Source: CAD feature listing. Evaluate the final solid. Frame: model axes, mm. A direction names the side the tool comes from. Give positions to 0.01 mm unless a question says otherwise; leave off trailing zeros. Order: outer loops, then holes, each group sorted by start corner. A loop starts at its lowest first (then second) coordinate and runs counter-clockwise, first axis right, second up.
1) Material intervals for line 1 (X direction, y = 3.75, z = 43); line 2 (X direction, y = 3, z = 8.5); line 3 (Z direction, x = 40.5, y = 27.25), sorted ascending.
2) Section C-C, the plane x = 43.5. Return loops of the section in (y, z), plus the area to 3 significant figures.
3) Section B-B, the plane z = 20. Return loops of the section in (x, y).
4) First-contact query: P1, Ø3, axis at y = 13.5, z = 16.5, coming from the +X side; P2, Ø2, axis at y = 13.5, z = 23.5, coming from the -X side; P3, Ø1, axis at x = 58, y = 11.5, coming from the -Z side; P4, Ø10, axis at y = 6.5, z = 9, coming from the -X side. Flat tips, straight axial feed; report the tip coordinate or a pass-through.
5) Access query for faces 1 (the face through (53, 23, 28.7)), 2 (the face through (60.25, 14, -2)), 3 (the face through (49.25, 14, 22)), 4 (the face through (21.75, 5, 27)). Directions: +Z, -Z, +X, -X, +Y, -Y. A direction counts if a zero-diameter tool reaches every point of the face in a straight line with its end or side. Return the directions, or none.
6) Section D-D, the plane x = 62. Return loops of the section in (y, z).
7) Draft query along X for faces 5 (the face through (49.25, 5, 27)), 6 (the face through (60.25, 5, 22)), 7 (the face through (55, 10.7, 23)). Return one class per face: released by +X, released by -X, zero draft, split by the parting line, or undercut.
8) Section A-A, the plane y = 6.5. Return loops of the section in (x, z), plus the area to 3 significant figures.
```python
from build123d import *

# Parameters (mm, degrees)
F0_W     = 10.75
F0_H     = 8.6
F1_DEPTH = 3.3
F0_W_2   = 27
F0_H_2   = 21
F0_W_3   = 7.25
F0_H_3   = 10.7
F0_H_4   = 6.6
F0_W_4   = 3.75
F2_DEPTH = 4.7
F3_DEPTH = 17.5
F4_DEPTH = 28.7
F5_DEPTH = 26
F6_DEPTH = 61.5
F7_SIZE  = 3
F8_R     = 1.5


with BuildPart() as f1:
    # F0 (on Top) → F1 (new body)
    with BuildSketch(Plane.XY):
        Polygon((-3.5, 0), (0, 0), (0, 8.6), (0, 9), (-3.5, 9), align=None)
        with Locations((5.375, 4.3)):
            Rectangle(F0_W, F0_H)
        Polygon((0, 9), (0, 8.6), (10.75, 8.6), (10.75, 10.7), (10.75, 17.3), (10.75, 28), (0, 28), (0, 19), align=None)
    extrude(amount=-F1_DEPTH)



with BuildPart() as f1b:
    # F0 (on Top) → F1, piece 2 (new body)
    with BuildSketch(Plane.XY):
        Polygon((71, 19.4), (71, 19), (74.5, 19), (74.5, 28), (71, 28), align=None)
        with Locations((65.625, 23.7)):
            Rectangle(F0_W, F0_H)
        Polygon((60.25, 10.7), (60.25, 0), (71, 0), (71, 9), (71, 19), (71, 19.4), (60.25, 19.4), (60.25, 17.3), align=None)
    extrude(amount=-F1_DEPTH)


with BuildPart() as f1_1:
    add(f1.part)

    add(f1b.part)  # F2 merges F1b
    # F0 (on Top) → F2 (join)
    with BuildSketch(Plane.XY):
        Polygon((21.75, 10.7), (21.75, 0), (49.25, 0), (49.25, 10.7), (49.25, 17.3), (49.25, 28), (21.75, 28), (21.75, 17.3), align=None)
        with Locations((35.5, 14)):
            Rectangle(F0_W_2, F0_H_2, mode=Mode.SUBTRACT)
        with Locations((35.5, 14)):
            Rectangle(F0_W_2, F0_H_2)
        Polygon((0, 9), (0, 8.6), (10.75, 8.6), (10.75, 10.7), (10.75, 17.3), (10.75, 28), (0, 28), (0, 19), align=None)
        Polygon((60.25, 10.7), (60.25, 0), (71, 0), (71, 9), (71, 19), (71, 19.4), (60.25, 19.4), (60.25, 17.3), align=None)
        with Locations((65.625, 23.7)):
            Rectangle(F0_W, F0_H)
        with Locations((5.375, 4.3)):
            Rectangle(F0_W, F0_H)
        with Locations((56.625, 5.35)):
            Rectangle(F0_W_3, F0_H_3)
        Polygon((53, 28), (53, 17.3), (60.25, 17.3), (60.25, 19.4), (60.25, 28), align=None)
        Polygon((10.75, 8.6), (10.75, 0), (18, 0), (18, 10.7), (10.75, 10.7), align=None)
        with Locations((14.375, 22.65)):
            Rectangle(F0_W_3, F0_H_3)
        with Locations((14.375, 14)):
            Rectangle(F0_W_3, F0_H_4)
        with Locations((56.625, 14)):
            Rectangle(F0_W_3, F0_H_4)
        with Locations((51.125, 5.35)):
            Rectangle(F0_W_4, F0_H_3)
        with Locations((19.875, 5.35)):
            Rectangle(F0_W_4, F0_H_3)
        with Locations((51.125, 22.65)):
            Rectangle(F0_W_4, F0_H_3)
        with Locations((19.875, 22.65)):
            Rectangle(F0_W_4, F0_H_3)
        Polygon((71, 19.4), (71, 19), (74.5, 19), (74.5, 28), (71, 28), align=None)
        Polygon((-3.5, 0), (0, 0), (0, 8.6), (0, 9), (-3.5, 9), align=None)
        with Locations((19.875, 14)):
            Rectangle(F0_W_4, F0_H_4)
        with Locations((51.125, 14)):
            Rectangle(F0_W_4, F0_H_4)
    extrude(amount=F2_DEPTH)

    # F0 (on Top) → F3 (join)
    with BuildSketch(Plane.XY):
        Polygon((0, 9), (0, 8.6), (10.75, 8.6), (10.75, 10.7), (10.75, 17.3), (10.75, 28), (0, 28), (0, 19), align=None)
        Polygon((60.25, 10.7), (60.25, 0), (71, 0), (71, 9), (71, 19), (71, 19.4), (60.25, 19.4), (60.25, 17.3), align=None)
        with Locations((14.375, 14)):
            Rectangle(F0_W_3, F0_H_4)
        with Locations((19.875, 14)):
            Rectangle(F0_W_4, F0_H_4)
        with Locations((51.125, 14)):
            Rectangle(F0_W_4, F0_H_4)
        with Locations((56.625, 14)):
            Rectangle(F0_W_3, F0_H_4)
    extrude(amount=F3_DEPTH)

    # F0 (on Top) → F4 (join)
    with BuildSketch(Plane.XY):
        with Locations((14.375, 22.65)):
            Rectangle(F0_W_3, F0_H_3)
        Polygon((10.75, 8.6), (10.75, 0), (18, 0), (18, 10.7), (10.75, 10.7), align=None)
        with Locations((19.875, 5.35)):
            Rectangle(F0_W_4, F0_H_3)
        with Locations((19.875, 22.65)):
            Rectangle(F0_W_4, F0_H_3)
        with Locations((51.125, 22.65)):
            Rectangle(F0_W_4, F0_H_3)
        Polygon((53, 28), (53, 17.3), (60.25, 17.3), (60.25, 19.4), (60.25, 28), align=None)
        with Locations((56.625, 5.35)):
            Rectangle(F0_W_3, F0_H_3)
        with Locations((51.125, 5.35)):
            Rectangle(F0_W_4, F0_H_3)
    extrude(amount=F4_DEPTH)

    # F0 (on Top) → F5 (join)
    with BuildSketch(Plane.XY):
        Polygon((21.75, 10.7), (21.75, 0), (49.25, 0), (49.25, 10.7), (49.25, 17.3), (49.25, 28), (21.75, 28), (21.75, 17.3), align=None)
        with Locations((35.5, 14)):
            Rectangle(F0_W_2, F0_H_2, mode=Mode.SUBTRACT)
    extrude(amount=F5_DEPTH)

    # F0 (on Top) → F6 (join)
    with BuildSketch(Plane.XY):
        with Locations((35.5, 14)):
            Rectangle(F0_W_2, F0_H_2)
    extrude(amount=F6_DEPTH)

    # F7
    f7_edges = [f1_1.edges().sort_by_distance(p)[0] for p in [
        (10.75, 22.65, 28.7),
        (10.75, 5.35, 28.7),
        (60.25, 5.35, 28.7),
        (60.25, 22.65, 28.7),
        (0, 18.3, 17.5),
        (71, 9.7, 17.5),
    ]]
    chamfer(f7_edges, length=F7_SIZE)

    # F8
    f8_edges = [f1_1.edges().sort_by_distance(p)[0] for p in [
        (-3.5, 0, 0.7),
        (74.5, 28, 0.7),
        (74.5, 19, 0.7),
        (-3.5, 9, 0.7),
    ]]
    fillet(f8_edges, radius=F8_R)


solid = f1_1.part
```
From the geometry:
1. line 1: x = 22 to 49
1. line 2: x = 10.75 to 71
1. line 3: z = 0 to 26
2. outline: (0, 0) - (28, 0) - (28, 26) - (24.5, 26) - (24.5, 61.5) - (3.5, 61.5) - (3.5, 26) - (0, 26) - close
2. area: 1,470 mm2
3. outline: (10.75, 0) - (60.25, 0) - (60.25, 10.7) - (49.25, 10.7) - (49.25, 17.3) - (60.25, 17.3) - (60.25, 28) - (10.75, 28) - (10.75, 17.3) - (21.75, 17.3) - (21.75, 10.7) - (10.75, 10.7) - close
4. P1: stops at x = 70.5
4. P2: stops at x = 21.75
4. P3: stops at z = 0
4. P4: stops at x = -3.5
5. face 1: +Z, +X, +Y, -Y
5. face 2: -Z, +Y, -Y
5. face 3: +Z, +X
5. face 4: +Z, +Y, -Y
6. outline: (0, -3.3) - (28, -3.3) - (28, 4.7) - (19.4, 4.7) - (19.4, 17.5) - (0, 17.5) - close
7. face 5: undercut
7. face 6: released by +X
7. face 7: zero draft
8. outline: (-3.5, -3.3) - (10.75, -3.3) - (10.75, 0) - (60.25, 0) - (60.25, -3.3) - (71, -3.3) - (71, 14.5) - (68, 17.5) - (60.25, 17.5) - (60.25, 25.7) - (57.25, 28.7) - (49.25, 28.7) - (49.25, 26) - (49, 26) - (49, 61.5) - (22, 61.5) - (22, 26) - (21.75, 26) - (21.75, 28.7) - (13.75, 28.7) - (10.75, 25.7) - (10.75, 4.7) - (-3.5, 4.7) - close
8. area: 2,630 mm2
